For this review, take the finished solid that the model builds, in its own axes (mm). A direction names the side the tool comes from. Coordinates: 2 decimals unless noted, no trailing zeros. Loops run counter-clockwise (first coordinate to the right, second up) from the corner with the lowest first, then second, coordinate; pieces in that order, holes last.
```python
from build123d import *

# Parameters (mm, degrees)
CUBE_W                    = 150
CUBE_H                    = 150
BOSS_EXTRU_1_DEPTH        = 34.5
PAVE_W                    = 96
PAVE_H                    = 144
ENL_V_MAT_EXTRU_1_DEPTH   = 31.5
VIS1_R                    = 2.5
ENL_V_MAT_EXTRU_2_DEPTH   = 5
ENL_V_START               = -5
VIS2_R                    = 2.5
ENL_V_MAT_EXTRU_3_DEPTH   = 5
PAVE_PROCHE_MOTEUR_W      = 12.5
PAVE_PROCHE_MOTEUR_H      = 124
ENL_V_MAT_EXTRU_4_DEPTH   = 31.5
PAVE_ROUE_LIBRE_W         = 32.86
PAVE_ROUE_LIBRE_H         = 15.696676457
PAVE_ROUE_LIBRE_H_2       = 18.419496328
ENL_V_MAT_EXTRU_5_DEPTH   = 36
CABLES_W                  = 22.36
CABLES_H                  = 10
ENL_V_MAT_EXTRU_6_DEPTH   = 36
ROUE_EXT_R                = 32
ENL_V_MAT_EXTRU_7_DEPTH   = 8
ROUE_INTER_R              = 16.02
ENL_V_MAT_EXTRU_8_DEPTH   = 69
ENL_V_START_2             = -7.5
ROUE_EXT2_R               = 32
ENL_V_MAT_EXTRU_9_DEPTH   = 7.5
ENL_V_START_3             = -69
ROUE_INTER2_R             = 16.02
ENL_V_MAT_EXTRU_10_DEPTH  = 69
VIS_MOTEUR_POUR_SUPPORT_R = 2.5
ENL_V_MAT_EXTRU_11_DEPTH  = 10
BOSS_EXTRU_2_DEPTH        = 10
ESQUISSE2_R               = 2.5
ENL_V_MAT_EXTRU_12_DEPTH  = 10
ESQUISSE3_W               = 3.439870431
ESQUISSE3_H               = 124
BOSS_EXTRU_3_DEPTH        = 31
ESQUISSE5_W               = 3.439870431
ESQUISSE5_H               = 124
BOSS_EXTRU_4_DEPTH        = 0.5
ESQUISSE6_R               = 2.5
ENL_V_MAT_EXTRU_13_DEPTH  = 10
ESQUISSE7_R               = 2.5
ENL_V_MAT_EXTRU_14_DEPTH  = 10
ESQUISSE8_R               = 2.5
ENL_V_MAT_EXTRU_15_DEPTH  = 10
ESQUISSE10_W              = 102.704284834
ESQUISSE10_H              = 150
ENL_V_MAT_EXTRU_16_DEPTH  = 40


with BuildPart() as part:
    # Cube → Boss.-Extru.1 (new body)
    with BuildSketch(Plane(origin=(0, 0, 0), x_dir=(1, 0, 0), z_dir=(0, 1, 0))):
        with Locations((-34.210526316, -11.513157895)):
            Rectangle(CUBE_W, CUBE_H)
    extrude(amount=BOSS_EXTRU_1_DEPTH)

    # Pave → Enlèv. mat.-Extru.1 (cut)
    with BuildSketch(Plane(origin=(0, 34.5, 0), x_dir=(1, 0, 0), z_dir=(0, 1, 0))):
        with Locations((-10.210526316, -11.513157895)):
            Rectangle(PAVE_W, PAVE_H)
    extrude(amount=-ENL_V_MAT_EXTRU_1_DEPTH, mode=Mode.SUBTRACT)

    # Vis1 → Enlèv. mat.-Extru.2 (cut)
    with BuildSketch(Plane.XY.offset(86.513157895)):
        with Locations((33.789473684, 10)):
            Circle(VIS1_R)
        with Locations((33.789473684, 20)):
            Circle(VIS1_R)
        with Locations((33.789473684, 30)):
            Circle(VIS1_R)
    extrude(amount=-ENL_V_MAT_EXTRU_2_DEPTH, mode=Mode.SUBTRACT)

    # Vis2 → Enlèv. mat.-Extru.3 (cut)
    with BuildSketch(Plane(origin=(0, 0, -63.486842105), x_dir=(-1, 0, 0), z_dir=(0, 0, -1)).offset(ENL_V_START)):
        with Locations(Location((-33.789473684, 10, 0), (0, 0, 180))):
            Circle(VIS2_R)
        with Locations(Location((-33.789473684, 20, 0), (0, 0, 180))):
            Circle(VIS2_R)
        with Locations(Location((-33.789473684, 30, 0), (0, 0, 180))):
            Circle(VIS2_R)
    extrude(amount=ENL_V_MAT_EXTRU_3_DEPTH, mode=Mode.SUBTRACT)

    # Pave proche moteur → Enlèv. mat.-Extru.4 (cut)
    with BuildSketch(Plane(origin=(0, 34.5, 0), x_dir=(1, 0, 0), z_dir=(0, 1, 0))):
        with Locations((-67.460526316, -11.513157895)):
            Rectangle(PAVE_PROCHE_MOTEUR_W, PAVE_PROCHE_MOTEUR_H)
    extrude(amount=-ENL_V_MAT_EXTRU_4_DEPTH, mode=Mode.SUBTRACT)

    # Pave Roue libre → Enlèv. mat.-Extru.5 (cut)
    with BuildSketch(Plane(origin=(0, 34.5, 0), x_dir=(1, 0, 0), z_dir=(0, 1, 0))):
        with Locations((-87.980526316, 61.335180334)):
            Rectangle(PAVE_ROUE_LIBRE_W, PAVE_ROUE_LIBRE_H)
        with Locations((-87.980526316, -85.722906059)):
            Rectangle(PAVE_ROUE_LIBRE_W, PAVE_ROUE_LIBRE_H_2)
    extrude(amount=-ENL_V_MAT_EXTRU_5_DEPTH, mode=Mode.SUBTRACT)

    # Cables → Enlèv. mat.-Extru.6 (cut)
    with BuildSketch(Plane(origin=(0, 34.5, 0), x_dir=(1, 0, 0), z_dir=(0, 1, 0))):
        with Locations((-89.710526316, -0.513157895)):
            Rectangle(CABLES_W, CABLES_H)
        with Locations((-89.710526316, -22.513157895)):
            Rectangle(CABLES_W, CABLES_H)
    extrude(amount=-ENL_V_MAT_EXTRU_6_DEPTH, mode=Mode.SUBTRACT)

    # Roue ext → Enlèv. mat.-Extru.7 (cut)
    with BuildSketch(Plane.XY.offset(86.513157895)):
        with Locations((-82.5, 10)):
            Circle(ROUE_EXT_R)
    extrude(amount=-ENL_V_MAT_EXTRU_7_DEPTH, mode=Mode.SUBTRACT)

    # Roue inter → Enlèv. mat.-Extru.8 (cut)
    with BuildSketch(Plane.XY.offset(86.513157895)):
        with Locations((-82.5, 10)):
            Circle(ROUE_INTER_R)
    extrude(amount=-ENL_V_MAT_EXTRU_8_DEPTH, mode=Mode.SUBTRACT)

    # Roue ext2 → Enlèv. mat.-Extru.9 (cut)
    with BuildSketch(Plane(origin=(0, 0, -63.486842105), x_dir=(-1, 0, 0), z_dir=(0, 0, -1)).offset(ENL_V_START_2)):
        with Locations((82.5, 10)):
            Circle(ROUE_EXT2_R)
    extrude(amount=ENL_V_MAT_EXTRU_9_DEPTH, mode=Mode.SUBTRACT)

    # Roue inter2 → Enlèv. mat.-Extru.10 (cut)
    with BuildSketch(Plane(origin=(0, 0, -63.486842105), x_dir=(-1, 0, 0), z_dir=(0, 0, -1)).offset(ENL_V_START_3)):
        with Locations((82.5, 10)):
            Circle(ROUE_INTER2_R)
    extrude(amount=ENL_V_MAT_EXTRU_10_DEPTH, mode=Mode.SUBTRACT)

    # Vis Moteur pour support → Enlèv. mat.-Extru.11 (cut)
    with BuildSketch(Plane(origin=(-58.210526316, 0, 0), x_dir=(0, 0, -1), z_dir=(1, 0, 0))):
        with Locations((-68.513157895, 8)):
            Circle(VIS_MOTEUR_POUR_SUPPORT_R)
        with Locations((-68.513157895, 18)):
            Circle(VIS_MOTEUR_POUR_SUPPORT_R)
        with Locations((-68.513157895, 28)):
            Circle(VIS_MOTEUR_POUR_SUPPORT_R)
        with Locations((45.986842105, 8)):
            Circle(VIS_MOTEUR_POUR_SUPPORT_R)
        with Locations((45.986842105, 18)):
            Circle(VIS_MOTEUR_POUR_SUPPORT_R)
        with Locations((45.986842105, 28)):
            Circle(VIS_MOTEUR_POUR_SUPPORT_R)
    extrude(amount=-ENL_V_MAT_EXTRU_11_DEPTH, mode=Mode.SUBTRACT)

    # Esquisse1 → Boss.-Extru.2 (add)
    with BuildSketch(Plane(origin=(0, 3, 0), x_dir=(1, 0, 0), z_dir=(0, 1, 0))):
        Polygon((-58.210526316, -15.513157895), (-14.210526316, -15.513157895), (-14.210526316, -83.513157895), (-6.210526316, -83.513157895), (-6.210526316, -15.513157895), (37.789473684, -15.513157895), (37.789473684, -7.513157895), (-6.210526316, -7.513157895), (-6.210526316, 60.486842105), (-14.210526316, 60.486842105), (-14.210526316, -7.513157895), (-58.210526316, -7.513157895), align=None)
    extrude(amount=BOSS_EXTRU_2_DEPTH)

    # Esquisse2 → Enlèv. mat.-Extru.12 (cut)
    with BuildSketch(Plane.XY.offset(15.513157895)):
        with Locations((-43.942882256, 8)):
            Circle(ESQUISSE2_R)
        with Locations((-26.88958752, 8)):
            Circle(ESQUISSE2_R)
        with Locations((9.588466595, 8)):
            Circle(ESQUISSE2_R)
        with Locations((23.56238511, 8)):
            Circle(ESQUISSE2_R)
    extrude(amount=-ENL_V_MAT_EXTRU_12_DEPTH, mode=Mode.SUBTRACT)

    # Esquisse3 → Boss.-Extru.3 (add)
    with BuildSketch(Plane(origin=(0, 3, 0), x_dir=(1, 0, 0), z_dir=(0, 1, 0))):
        with Locations((-62.930461532, -11.513157895)):
            Rectangle(ESQUISSE3_W, ESQUISSE3_H)
    extrude(amount=BOSS_EXTRU_3_DEPTH)

    # Esquisse5 → Boss.-Extru.4 (add)
    with BuildSketch(Plane(origin=(0, 34, 0), x_dir=(1, 0, 0), z_dir=(0, 1, 0))):
        with Locations((-62.930461532, -11.513157895)):
            Rectangle(ESQUISSE5_W, ESQUISSE5_H)
    extrude(amount=BOSS_EXTRU_4_DEPTH)

    # Esquisse6 → Enlèv. mat.-Extru.13 (cut)
    with BuildSketch(Plane(origin=(-58.210526316, 0, 0), x_dir=(0, 0, -1), z_dir=(1, 0, 0))):
        with Locations((-68.513157895, 28)):
            Circle(ESQUISSE6_R)
        with Locations((-68.513157895, 18)):
            Circle(ESQUISSE6_R)
        with Locations((-68.513157895, 8)):
            Circle(ESQUISSE6_R)
        with Locations((45.986842105, 28)):
            Circle(ESQUISSE6_R)
        with Locations((45.986842105, 18)):
            Circle(ESQUISSE6_R)
        with Locations((45.986842105, 8)):
            Circle(ESQUISSE6_R)
    extrude(amount=-ENL_V_MAT_EXTRU_13_DEPTH, mode=Mode.SUBTRACT)

    # Esquisse7 → Enlèv. mat.-Extru.14 (cut)
    with BuildSketch(Plane(origin=(-58.210526316, 0, 0), x_dir=(0, 0, -1), z_dir=(1, 0, 0))):
        with Locations((0, 8.527871685)):
            Circle(ESQUISSE7_R)
        with Locations((0, 18.750861141)):
            Circle(ESQUISSE7_R)
        with Locations((-25.400224022, 8.527871685)):
            Circle(ESQUISSE7_R)
        with Locations((-25.400224022, 18.750861141)):
            Circle(ESQUISSE7_R)
        with Locations((-50.386538843, 8.527871685)):
            Circle(ESQUISSE7_R)
        with Locations((23.629525814, 8.527871685)):
            Circle(ESQUISSE7_R)
    extrude(amount=-ENL_V_MAT_EXTRU_14_DEPTH, mode=Mode.SUBTRACT)

    # Esquisse8 → Enlèv. mat.-Extru.15 (cut)
    with BuildSketch(Plane(origin=(0, 3, 0), x_dir=(1, 0, 0), z_dir=(0, 1, 0))):
        with Locations(Location((19.789473684, -43.513157895, 0), (0, 0, 270))):
            Circle(ESQUISSE8_R)
        with Locations(Location((19.789473684, 20.486842105, 0), (0, 0, 270))):
            Circle(ESQUISSE8_R)
    extrude(amount=-ENL_V_MAT_EXTRU_15_DEPTH, mode=Mode.SUBTRACT)

    # Esquisse10 → Enlèv. mat.-Extru.16 (cut)
    with BuildSketch(Plane(origin=(0, 34.5, 0), x_dir=(1, 0, 0), z_dir=(0, 1, 0))):
        with Locations((-10.562668733, -11.513157895)):
            Rectangle(ESQUISSE10_W, ESQUISSE10_H)
    extrude(amount=-ENL_V_MAT_EXTRU_16_DEPTH, mode=Mode.SUBTRACT)


solid = part.part
```
Q1. For pin 1 Ø4.5 at (y, z) = (28, 68.51) entering from +X; pin 2 Ø3 at (x, y) = (-66, 12) entering from -Z; pin 3 Ø5 at (y, z) = (25.5, -59.5) entering from +X; pin 4 Ø8 at (y, z) = (8.53, 0) entering from +X, all flat-tipped, find the tip position at first contact; note any pin that passes through.
Q2. Consider section B-B (z = 0). State the section outline as (x, y) points.
Q3. The part is to be moulded in two halves that separate along Z. For faces 5 (the face through (-104.411, 18.6, -55.5)), 6 (the face through (-107, 33, 86.513)), 7 (the face through (-63.26, 20.86, -1.34)), say which applies: +Z half, -Z half, draft (parallel to the pull), parting line (faces both ways), or undercut.
Q4. Machinability: for faces 1 (the face through (-63.26, 6.48, 70.5)), 2 (the face through (-71.551, 28, -55)), 3 (the face through (-66, 21, -55.987)), 4 (the face through (-66, 21, 78.513)), which of the approach directions +Z, -Z, +X, -X, +Y, -Y give a long, thin tool a straight path to every point of the face, cutting with its end or side? Answer none if there is none.
Q5. Consider section A-A (x = -82.5). State the section outline as (y, z) points.
Q6. Consider section D-D (x = -75). State the section outline as (y, z) points.
Q7. Wall thickness on probe 1 along X at (y, z) = (31, -32); probe 2 along Z at (x, y) = (-65, 23); probe 3 along X at (y, z) = (10, -32): over which ranges is each line inside the solid? List them lowest first.
Q8. Consider section C-C (z = 55). State the section outline as (x, y) points.
Model answer:
1. pin 1: stops at x = -73.71
1. pin 2: stops at z = -55.99
1. pin 3: stops at x = -108.96
1. pin 4: stops at x = -61.91
2. outline: (-109.21, 0) - (-100.89, 0) - (-100.89, 34.5) - (-109.21, 34.5) - close; (-78.53, 25.52) arc R16.02 cw to (-73.71, 23.39) - (-73.71, 34.5) - (-78.53, 34.5) - close; (-69.98, 0) - (-61.91, 0) - (-61.91, 6.03) - (-64.65, 6.03) - (-64.65, 3) - (-68.09, 3) arc R16.02 cw to start; (-64.65, 11.03) - (-61.91, 11.03) - (-61.91, 16.25) - (-64.65, 16.25) - close; (-64.65, 21.25) - (-61.91, 21.25) - (-61.91, 34.5) - (-64.65, 34.5) - close
3. face 5: draft
3. face 6: +Z half
3. face 7: undercut
4. face 1: +X
4. face 2: -Z, +Y, -Y
4. face 3: -Z, +X, +Y, -Y
4. face 4: +Z, +X, +Y, -Y
5. outline: (0, 5.51) - (34.5, 5.51) - (34.5, 17.51) - (0, 17.51) - close; (26.02, -53.49) - (34.5, -53.49) - (34.5, -4.49) - (26.02, -4.49) - close; (26.02, 27.51) - (34.5, 27.51) - (34.5, 76.51) - (26.02, 76.51) - close
6. outline: (0, 5.51) - (24.16, 5.51) - (24.16, -53.49) - (34.5, -53.49) - (34.5, 76.51) - (24.16, 76.51) - (24.16, 17.51) - (0, 17.51) - close
7. probe 1: x = -109.21 to -73.71, -64.65 to -61.91
7. probe 2: z = -55.99 to -50.49, 73.51 to 78.51
7. probe 3: x = -109.21 to -98.52, -64.65 to -61.91
8. outline: (-109.21, 0) - (-95.02, 0) arc R16.02 cw to (-73.71, 23.39) - (-73.71, 34.5) - (-109.21, 34.5) - close; (-69.98, 0) - (-61.91, 0) - (-61.91, 34.5) - (-64.65, 34.5) - (-64.65, 3) - (-68.09, 3) arc R16.02 cw to start
